from build123d import *

# Parameters (mm, degrees)
IZIM1_W                          = 60
IZIM1_H                          = 116
Y_KSEKLIK_EKSTR_ZYON1_DEPTH      = 60
IZIM2_R                          = 8
Y_KSEKLIK_EKSTR_ZYON2_DEPTH      = 9
IZIM3_R                          = 30
Y_KSEKLIK_EKSTR_ZYON3_DEPTH      = 60
IZIM4_R                          = 20
KES_EKSTR_ZYON1_DEPTH            = 20
IZIM5_R                          = 15
KES_EKSTR_ZYON2_DEPTH            = 20
IZIM6_R                          = 9
KES_EKSTR_ZYON3_DEPTH            = 20
IZIM7_R                          = 12
KES_EKSTR_ZYON4_DEPTH            = 20
IZIM8_R                          = 7
KES_EKSTR_ZYON5_DEPTH            = 25
IZIM9_R                          = 12
KES_EKSTR_ZYON6_DEPTH            = 15
KES_EKSTR_ZYON8_DEPTH            = 30
IZIM13_W                         = 60
IZIM13_H                         = 30
KES_EKSTR_ZYON9_DEPTH            = 30
IZIM14_R                         = 8
IZIM14_R_2                       = 4
Y_KSEKLIK_EKSTR_ZYON5_DEPTH      = 6
Y_KSEKLIK_EKSTR_ZYON5_DEPTH_BACK = 15
IZIM16_W                         = 8
IZIM16_H                         = 21
KES_EKSTR_ZYON10_DEPTH           = 57
KES_EKSTR_ZYON12_DEPTH           = 15
IZIM18_W                         = 42
IZIM18_H                         = 36
KES_EKSTR_ZYON13_DEPTH           = 18
Y_KSEKLIK_EKSTR_ZYON7_DEPTH      = 42


with BuildPart() as part:
    # Çizim1 → Yükseklik-Ekstrüzyon1 (new body)
    with BuildSketch(Plane(origin=(0, 0, 0), x_dir=(0, 0, -1), z_dir=(1, 0, 0))):
        with Locations((-30, 58)):
            Rectangle(IZIM1_W, IZIM1_H)
    extrude(amount=Y_KSEKLIK_EKSTR_ZYON1_DEPTH)

    # Çizim2 → Yükseklik-Ekstrüzyon2 (add)
    with BuildSketch(Plane(origin=(0, 0, 0), x_dir=(1, 0, 0), z_dir=(0, 1, 0))):
        with BuildLine():
            Line((57, 10), (3, 10))
            ThreePointArc((3, 10), (-19.192388155, 19.192388155), (-10, -3))
            Line((-10, -3), (-10, -57))
            ThreePointArc((-10, -57), (-19.192388155, -79.192388155), (3, -70))
            Line((3, -70), (57, -70))
            ThreePointArc((57, -70), (79.192388155, -79.192388155), (70, -57))
            Line((70, -57), (70, -3))
            ThreePointArc((70, -3), (79.192388155, 19.192388155), (57, 10))
        make_face()
        with Locations((-10, 10)):
            Circle(IZIM2_R, mode=Mode.SUBTRACT)
        with Locations((-10, -70)):
            Circle(IZIM2_R, mode=Mode.SUBTRACT)
        with Locations((70, -70)):
            Circle(IZIM2_R, mode=Mode.SUBTRACT)
        with Locations((70, 10)):
            Circle(IZIM2_R, mode=Mode.SUBTRACT)
    extrude(amount=-Y_KSEKLIK_EKSTR_ZYON2_DEPTH)

    # Çizim3 → Yükseklik-Ekstrüzyon3 (add)
    with BuildSketch(Plane.XY):
        with Locations((30, 116)):
            Circle(IZIM3_R)
    extrude(amount=Y_KSEKLIK_EKSTR_ZYON3_DEPTH)

    # Çizim4 → Kes-Ekstrüzyon1 (cut)
    with BuildSketch(Plane.XY.offset(60)):
        with Locations((30, 116)):
            Circle(IZIM4_R)
    extrude(amount=-KES_EKSTR_ZYON1_DEPTH, mode=Mode.SUBTRACT)

    # Çizim5 → Kes-Ekstrüzyon2 (cut)
    with BuildSketch(Plane.XY.offset(40)):
        with Locations((30, 116)):
            Circle(IZIM5_R)
    extrude(amount=-KES_EKSTR_ZYON2_DEPTH, mode=Mode.SUBTRACT)

    # Çizim6 → Kes-Ekstrüzyon3 (cut)
    with BuildSketch(Plane.XY.offset(20)):
        with Locations((30, 116)):
            Circle(IZIM6_R)
    extrude(amount=-KES_EKSTR_ZYON3_DEPTH, mode=Mode.SUBTRACT)

    # Çizim7 → Kes-Ekstrüzyon4 (cut)
    with BuildSketch(Plane.XY.offset(60)):
        with Locations((30, 36)):
            Circle(IZIM7_R)
    extrude(amount=-KES_EKSTR_ZYON4_DEPTH, mode=Mode.SUBTRACT)

    # Çizim8 → Kes-Ekstrüzyon5 (cut)
    with BuildSketch(Plane.XY.offset(40)):
        with Locations((30, 36)):
            Circle(IZIM8_R)
    extrude(amount=-KES_EKSTR_ZYON5_DEPTH, mode=Mode.SUBTRACT)

    # Çizim9 → Kes-Ekstrüzyon6 (cut)
    with BuildSketch(Plane.XY.offset(15)):
        with Locations((30, 36)):
            Circle(IZIM9_R)
    extrude(amount=-KES_EKSTR_ZYON6_DEPTH, mode=Mode.SUBTRACT)

    # Çizim10 → Kes-Ekstrüzyon8 (cut)
    with BuildSketch(Plane(origin=(60, 0, 0), x_dir=(0, 0, -1), z_dir=(1, 0, 0))):
        Polygon((-60, 116), (-60, 36), (-51, 36), (-9, 36), (0, 36), (0, 116), align=None)
    extrude(amount=-KES_EKSTR_ZYON8_DEPTH, mode=Mode.SUBTRACT)

    # Çizim13 → Kes-Ekstrüzyon9 (cut)
    with BuildSketch(Plane(origin=(30, 0, 0), x_dir=(0, 0, -1), z_dir=(1, 0, 0))):
        with Locations((-30, 131)):
            Rectangle(IZIM13_W, IZIM13_H)
    extrude(amount=KES_EKSTR_ZYON9_DEPTH, mode=Mode.SUBTRACT)

    # Çizim14 → Yükseklik-Ekstrüzyon5 (add, two sides)
    with BuildSketch(Plane(origin=(0, 146, 0), x_dir=(1, 0, 0), z_dir=(0, 1, 0))) as y_kseklik_ekstr_zyon5_sk:
        with Locations((30, -30)):
            Circle(IZIM14_R)
        with Locations((30, -30)):
            Circle(IZIM14_R_2, mode=Mode.SUBTRACT)
    extrude(amount=Y_KSEKLIK_EKSTR_ZYON5_DEPTH)
    extrude(y_kseklik_ekstr_zyon5_sk.sketch, amount=-Y_KSEKLIK_EKSTR_ZYON5_DEPTH_BACK)

    # Çizim16 → Kes-Ekstrüzyon10 (cut)
    with BuildSketch(Plane.XY.offset(46)):
        with Locations((34, 141.5)):
            Rectangle(IZIM16_W, IZIM16_H)
    extrude(amount=-KES_EKSTR_ZYON10_DEPTH, mode=Mode.SUBTRACT)

    # Çizim17 → Kes-Ekstrüzyon12 (cut)
    with BuildSketch(Plane(origin=(0, 146, 0), x_dir=(1, 0, 0), z_dir=(0, 1, 0))):
        with BuildLine():
            Line((30, -26), (30, -34))
            ThreePointArc((30, -34), (26, -30), (30, -26))
        make_face()
    extrude(amount=-KES_EKSTR_ZYON12_DEPTH, mode=Mode.SUBTRACT)

    # Çizim18 → Kes-Ekstrüzyon13 (cut)
    with BuildSketch(Plane(origin=(60, 0, 0), x_dir=(0, 0, -1), z_dir=(1, 0, 0))):
        with Locations((-30, 18)):
            Rectangle(IZIM18_W, IZIM18_H)
    extrude(amount=-KES_EKSTR_ZYON13_DEPTH, mode=Mode.SUBTRACT)

    # Çizim21 → Yükseklik-Ekstrüzyon7 (add)
    with BuildSketch(Plane(origin=(0, 0, 51), x_dir=(-1, 0, 0), z_dir=(0, 0, -1))):
        with BuildLine():
            Line((-42, 29), (-42, 36))
            Line((-42, 36), (-49, 36))
            ThreePointArc((-49, 36), (-46.949747468, 31.050252532), (-42, 29))
        make_face()
    extrude(amount=Y_KSEKLIK_EKSTR_ZYON7_DEPTH)


solid = part.part
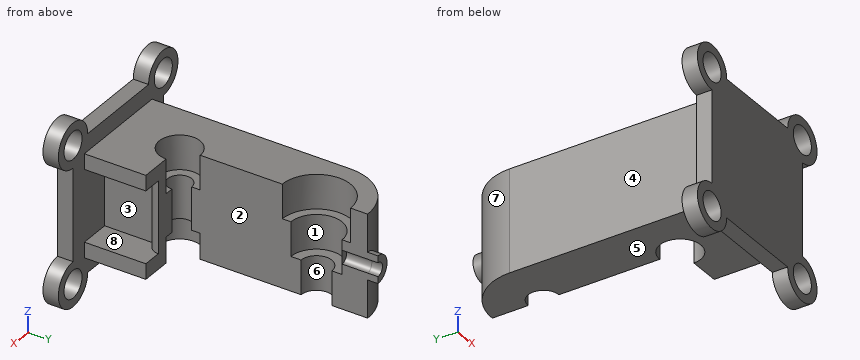
Input: part model. Units: mm. Frame: model coordinates. Face numbers are marked on the shaded views. A direction names the side the tool comes from. Give positions to 0.01 mm unless a question says otherwise; leave off trailing zeros. Order: outer loops, then holes, each group sorted by start corner. A loop starts at its lowest first (then second) coordinate and runs counter-clockwise, first axis right, second up. Notation, with made-up numbers: (73.25, 54.25) - (120.25, 54.25) arc R23 cw to (120.25, 79.25) - close; hole circle Ø5 at (-36.5, -31). An arc over 180 degrees is marked (long way). Write each question's results on one line, items separated by ' | '.
Item 1: Material intervals for line 1 along Y through (x, z) = (60, -15); line 2 along X through (y, z) = (48.5, 10.5); line 3 along Z through (x, y) = (59.5, 7), sorted ascending.
A:
line 1: y = -9 to 0 | line 2: x = 0 to 30 | line 3: z = 0 to 9, 51 to 60
Item 2: Section B-B (x = 72). Return loops of the section in (y, z), and give its area (3 significant figures).
A:
outline: (-9, -22.85) - (0, -22.85) - (0, -17.75) - (-9, -17.75) - close; (-9, -2.25) - (0, -2.25) - (0, 2.85) - (-9, 2.85) - close; (-9, 57.15) - (0, 57.15) - (0, 62.25) - (-9, 62.25) - close; (-9, 77.75) - (0, 77.75) - (0, 82.85) - (-9, 82.85) - close | area: 184 mm^2
Item 3: Section D-D (z = 45). Return loops of the section in (x, y), and give its area (3 significant figures).
A:
outline: (-10, -9) - (70, -9) - (70, 0) - (42, 0) - (42, 29) arc R7 ccw to (49, 36) - (42, 36) arc R12 cw (long way) to (30, 48) - (30, 96) arc R20 cw to (30, 136) - (30, 146) arc R30 ccw to (0, 116) - (0, 0) - (-10, 0) - close | area: 4,410 mm^2
Item 4: Access query for the marked faces 1, 2, 3 and 4. Directions: +Z, -Z, +X, -X, +Y, -Y. A direction counts if a zero-diameter tool reaches every point of the face in a straight line with its end or side. Return the directions, or none.
A:
face 1: +Z, +X | face 2: +Z, -Z, +X, +Y | face 3: +X | face 4: +Z, -Z, -X, +Y
Item 5: Draft query along Y for the marked faces 5, 6, 7 and 8. Return one class per face: released by +Y, released by -Y, zero draft, split by the parting line, or undercut.
A:
face 5: zero draft | face 6: undercut | face 7: released by +Y | face 8: undercut
Item 6: Contact query for flat-ended pins moving along their axis: pin 1 Ø3 at (x, z) = (15, 42.5) entering from +Y; pin 2 Ø19 at (x, y) = (29, 40) entering from +Z; pin 3 Ø4.5 at (y, z) = (-2.5, 26.5) entering from +X. Output: stop coordinate, or through.
A:
pin 1: stops at y = 142.79 | pin 2: stops at z = 60 | pin 3: stops at x = 70
Item 7: Section C-C (y = 19). Return loops of the section in (x, z), and give its area (3 significant figures).
A:
outline: (0, 0) - (60, 0) - (60, 9) - (42, 9) - (42, 51) - (60, 51) - (60, 60) - (0, 60) - close | area: 2,840 mm^2
Item 8: Section A-A (z = -7). Return loops of the section in (x, y).
A:
outline: (-22.65, -9) - (-17.42, -9) - (-17.42, 0) - (-22.65, 0) - close; (-2.58, -9) - (62.58, -9) - (62.58, 0) - (-2.58, 0) - close; (77.42, -9) - (82.65, -9) - (82.65, 0) - (77.42, 0) - close
